```python
from build123d import *

# Parameters (mm, degrees)
F0_R     = 8
F1_DEPTH = 1.5
F3_DEPTH = 2.4
F4_T     = -1.2
F5_R     = 1.49999


# Not quite as in the source:
# - a fillet or chamfer is up to 0.001 mm smaller than in the source, because OpenCascade refuses the exact size


with BuildPart() as f1:
    # F0 (on Top) → F1 (new body)
    with BuildSketch(Plane.XY):
        Circle(F0_R)
    extrude(amount=F1_DEPTH)

    # F2 (on face) → F3 (join)
    with BuildSketch(Plane.XY.offset(1.5)):
        Polygon((5.8, -3.3486315613), (5.8, 3.3486315613), (0, 6.6972631226), (-5.8, 3.3486315613), (-5.8, -3.3486315613), (0, -6.6972631226), align=None)
    extrude(amount=F3_DEPTH)

    # F4
    f4_openings = [f1.faces().sort_by_distance(p)[0] for p in [
        (0, 0, 3.9),
    ]]
    offset(amount=F4_T, openings=f4_openings, kind=Kind.INTERSECTION)

    # F5 (radius 1.5 in the source; OpenCascade refuses exactly that, so slightly less here)
    f5_edges = [f1.edges().sort_by_distance(p)[0] for p in [
        (-8, 0, 0),
    ]]
    fillet(f5_edges, radius=F5_R)


solid = f1.part
```
Geometry: final body of the model. Coordinates: model frame, mm. A direction names the side the tool comes from. Coordinates: 2 decimals unless noted, no trailing zeros. Order: outer loops, then holes, each group sorted by start corner. A loop starts at its lowest first (then second) coordinate and runs counter-clockwise, first axis right, second up. Notation, with made-up numbers: (-24, -34.75) - (-7, -34.75) arc R31 ccw to (-7, 4.25) - close; hole circle Ø10 at (-37, 5). An arc over 180 degrees is marked (long way). Return JSON: item names as keys, results as strings. Group by question number.
1. Pin query (flat end, axial travel): pin 1 (2 mm diameter, centred on x = -6.5, z = 3, fed in from +Y); pin 2 (1.4 mm diameter, centred on y = -1, z = 2.5, fed in from +X). Return the tip coordinate at first contact, or that it passes through.
2. Set-up query: faces 4 (the face through (-2.94, -5, 2.68)), 5 (the face through (-5.8, 0, 3)), 6 (the face through (4, -5, 1.5)), 7 (the face through (5.8, 0, 3)). Return all of +Z, -Z, +X, -X, +Y, -Y with unobstructed straight access to the full face (end or side cutting, diameter ignored); none if empty.
3. Cut plane A-A (z = 3.05). Output: boundary loops of the cut face in (x, y).
4. Material intervals for line 1 along X through (y, z) = (-2.5, 3.15); line 2 along Z through (x, y) = (6, 1.5); line 3 along X through (y, z) = (5, 1.9), sorted ascending. Write a range as [from, to].
5. Pull-direction query (X, two-part tool) for faces 1 (the face through (0, 0, 0)), 2 (the face through (0, 0, 1.2)), 3 (the face through (2.859, -5.046, 2.683)); classes: pulls with the +X half, pulls with the -X half, needs draft (parallel to the pull), parting line crosses it, or undercut.
Resolved:
{
 "1": {"pin 1": "stops at y = 3.52", "pin 2": "stops at x = 5.8"},
 "2": {"face 4": "+Z, -X, -Y", "face 5": "+Z, -X, +Y, -Y", "face 6": "+Z", "face 7": "+Z, +X, +Y, -Y"},
 "3": {"outline": "(-5.8, -3.35) - (0, -6.7) - (5.8, -3.35) - (5.8, 3.35) - (0, 6.7) - (-5.8, 3.35) - close; hole (-4.6, -2.66) - (0, -5.31) - (4.6, -2.66) - (4.6, 2.66) - (0, 5.31) - (-4.6, 2.66) - close"},
 "4": {"line 1": "x = [-5.8, -4.6], [4.6, 5.8]", "line 2": "z = [0, 1.5]", "line 3": "x = [-2.94, -0.54], [0.54, 2.94]"},
 "5": {"face 1": "needs draft", "face 2": "undercut", "face 3": "pulls with the +X half"}
}
